The figure shows three views and two pictorial views of one solid part (mm, origin at its lowest corner). Answer the questions. A direction names the side the tool comes from. Coordinates: 2 decimals unless noted, no trailing zeros. Order: outer loops, then holes, each group sorted by start corner. A loop starts at its lowest first (then second) coordinate and runs counter-clockwise, first axis right, second up. Notation, with made-up numbers: (47.25, -13) - (101.25, -13) arc R26 ccw to (101.25, 13) - close; hole circle Ø3 at (24, 60.5). An arc over 180 degrees is marked (long way). Use one line per item in the form item = value.
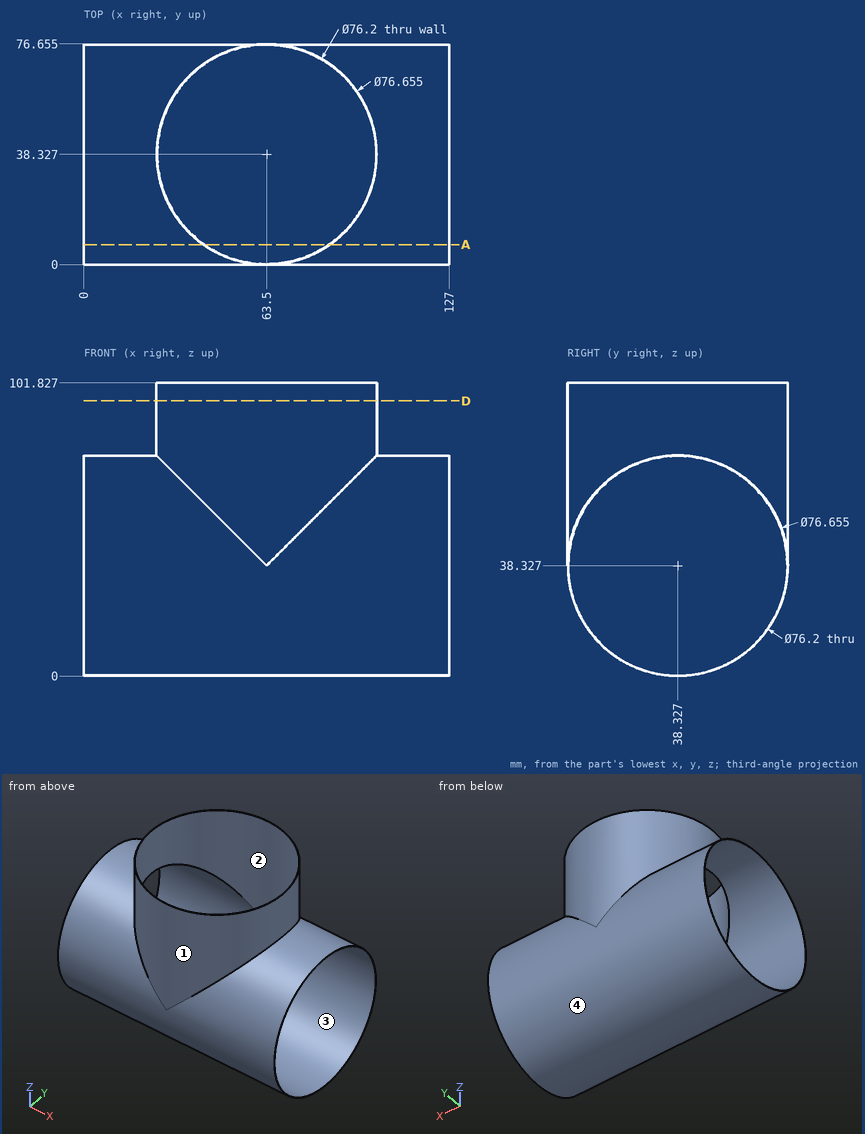
(1) Section D-D, the plane z = 95.5 is taken. Write down the section's boundary in (x, y) (1 decimal).
Answer list:
outline = circle Ø76.7 at (63.5, 38.3); hole circle Ø76.2 at (63.5, 38.3)
(2) Straight lines are drawn through the part: L1, parallel to Y at x = 63.5, z = 67 (1 decimal); L2, parallel to Y at x = 63, z = 66; L3, parallel to Z at x = 48.5, y = 38. For each, find the intervals that lie inside material, in ascending order.
Answer list:
L1 = 0 to 0.2, 76.4 to 76.7
L2 = 0 to 0.23, 76.42 to 76.65
L3 = 0 to 0.23
(3) Which of the six approach directions +Z, -Z, +X, -X, +Y, -Y give full straight-line access (tool end or side, diameter ignored) to the marked faces 3 and 4?
Answer list:
face_3 = +X, -X
face_4 = none
(4) The mould has two halves that part along X. Classify the marked faces 1 and 2: +X half, -X half, draft (parallel to the pull), parting line (faces both ways), or undercut.
Answer list:
face_1 = parting line
face_2 = undercut
(5) Section A-A, the plane y = 7 is taken. Write down the section's boundary in (x, z).
Answer list:
outline = (0, 16.25) - (127, 16.25) - (127, 16.64) - (0, 16.64) - close; (0, 60.01) - (41.82, 60.01) - (41.82, 101.83) - (41.42, 101.83) - (41.42, 60.41) - (0, 60.41) - close; (85.18, 60.01) - (127, 60.01) - (127, 60.41) - (85.58, 60.41) - (85.58, 101.83) - (85.18, 101.83) - close
(6) Given pin 1 Ø5 at (y, z) = (12, 15.5) entering from +X; pin 2 Ø6 at (y, z) = (25.5, 89) entering from +X; pin 3 Ø5 at (x, y) = (85.5, 34) entering from -Z; pin 4 Ø12 at (x, z) = (77, 52) entering from +Y, each flat-ended and moving along its own axis, determine where each tip first touches the part or whether it passes through.
Answer list:
pin_1 = through
pin_2 = 100.55
pin_3 = 0.04
pin_4 = 75.91
